Geometry: final body of the model. Coordinates: model frame, mm. A direction names the side the tool comes from. Round coordinates to 2 decimals unless told otherwise and drop trailing zeros. Loops run counter-clockwise (first coordinate to the right, second up) from the corner with the lowest first, then second, coordinate; pieces in that order, holes last. Notation, with made-up numbers: M 35.25,89.25 L 64.25,89.25 A20 cw 64.25,121.25 Z; hole C 50.25,7 d9. An arc over 180 degrees is marked long. Write each question's results on one line, items separated by ' | '.
```python
from build123d import *

# Parameters (mm, degrees)
F0_R     = 7.9375
F1_DEPTH = 0.79375
F3_DEPTH = 3.175
F4_R     = 0.79375
F6_D     = 6.35
F6_DEPTH = 19.05
F6_TIP   = 1.9077324654


with BuildPart() as f1:
    # F0 (on Top) → F1 (new body)
    with BuildSketch(Plane.XY):
        Circle(F0_R)
    extrude(amount=F1_DEPTH)

    # F2 (on face) → F3 (join)
    with BuildSketch(Plane.XY.offset(0.79375)):
        Polygon((-5.715, 2.367230509), (-5.715, -2.367230509), (-2.367230509, -5.715), (2.367230509, -5.715), (5.715, -2.367230509), (5.715, 2.367230509), (2.367230509, 5.715), (-2.367230509, 5.715), align=None)
    extrude(amount=F3_DEPTH)

    # F4
    f4_edges = [f1.edges().sort_by_distance(p)[0] for p in [
        (-5.715, -2.367231, 2.38125),
        (-2.367231, -5.715, 2.38125),
        (2.367231, -5.715, 2.38125),
        (5.715, -2.367231, 2.38125),
        (5.715, 2.367231, 2.38125),
        (2.367231, 5.715, 2.38125),
        (-2.367231, 5.715, 2.38125),
        (-5.715, 2.367231, 2.38125),
        (-4.041115, 4.041115, 0.79375),
        (0, 5.715, 0.79375),
        (-5.715, 0, 0.79375),
        (-4.041115, -4.041115, 0.79375),
        (0, -5.715, 0.79375),
        (4.041115, -4.041115, 0.79375),
        (5.715, 0, 0.79375),
        (4.041115, 4.041115, 0.79375),
    ]]
    fillet(f4_edges, radius=F4_R)

    # F6
    with Locations(Plane.XY.offset(3.96875)):
        with Locations((0, 0)):
            Hole(F6_D / 2, depth=F6_DEPTH)
            with Locations((0, 0, -(F6_DEPTH + F6_TIP / 2))):  # 118° drill point
                Cone(0, F6_D / 2, F6_TIP, mode=Mode.SUBTRACT)


solid = f1.part
```
1. Pin query (flat end, axial travel): P1, Ø1.2, axis at y = 0.5, z = 3, coming from the -X side (3 decimals); P2, Ø1.5, axis at x = 1.5, z = 2.5, coming from the +Y side (3 decimals); P3, Ø4, axis at x = 0, y = 0, coming from the -Z side; P4, Ø1.2, axis at x = 0, z = 2, coming from the -Y side. Return the tip coordinate at first contact, or that it passes through.
Answer key:
P1: stops at x = -5.715 | P2: stops at y = 5.715 | P3: passes through | P4: stops at y = -5.74
2. Ray query, probe 1 along Y at (x, z) = (0, 2.7) (3 decimals); probe 2 along Z at (x, y) = (2, -7); probe 3 along Y at (x, z) = (1, 0.7). Return the intervals inside material, ascending.
Answer key:
probe 1: y = -5.715 to -3.175, 3.175 to 5.715 | probe 2: z = 0 to 0.79 | probe 3: y = -7.87 to -3.01, 3.01 to 7.87
3. Draft query along X for faces 5 (the face through (-4.06, -4.02, 2.76)), 6 (the face through (0, -5.715, 3)), 7 (the face through (0.69, -3.1, 1.96)). Return one class per face: pulls with the +X half, pulls with the -X half, needs draft (parallel to the pull), parting line crosses it, or undercut.
Answer key:
face 5: pulls with the -X half | face 6: needs draft | face 7: undercut
4. Section D-D (z = 1.4). Output: boundary loops of the cut face in (x, y) (3 decimals), then the cut area to 3 significant figures.
Answer key:
outline: M -5.737,-2.038 A0.816 ccw -5.498,-2.616 L -2.616,-5.498 A0.816 ccw -2.038,-5.737 L 2.038,-5.737 A0.816 ccw 2.616,-5.498 L 5.498,-2.616 A0.816 ccw 5.737,-2.038 L 5.737,2.038 A0.816 ccw 5.498,2.616 L 2.616,5.498 A0.816 ccw 2.038,5.737 L -2.038,5.737 A0.816 ccw -2.616,5.498 L -5.498,2.616 A0.816 ccw -5.737,2.038 Z; hole C 0,0 d6.35 | area: 77.3 mm²
5. Access query for faces 1 (the face through (5.715, 0, 3)), 2 (the face through (-4.02, 4.06, 2.76)), 3 (the face through (4.02, -4.06, 2.76)), 4 (the face through (-5, 5, 0.794)). Directions: +Z, -Z, +X, -X, +Y, -Y. A direction counts if a zero-diameter tool reaches every point of the face in a straight line with its end or side. Return the directions, or none.
Answer key:
face 1: +Z, +X, +Y, -Y | face 2: +Z, -X, +Y | face 3: +Z, +X, -Y | face 4: +Z
6. Section B-B (y = 0). Output: boundary loops of the cut face in (x, z) (1 decimal).
Answer key:
outline: M -7.9,0 L -3.2,0 L -3.2,4 L -5.7,4 L -5.7,1.6 A0.8 cw -6.5,0.8 L -7.9,0.8 Z; M 3.2,0 L 7.9,0 L 7.9,0.8 L 6.5,0.8 A0.8 cw 5.7,1.6 L 5.7,4 L 3.2,4 Z
